Input: part model. Units: mm. Frame: model coordinates. A direction names the side the tool comes from. Coordinates: 2 decimals unless noted, no trailing zeros. Write each loop counter-clockwise with the first axis right and the second up, starting at its lowest first coordinate (ties: lowest second). Pieces come first, ordered by that corner, then holes.
from build123d import *

# Parameters (mm, degrees)
F0_W      = 14
F0_H      = 3
F0_W_2    = 3
F1_DEPTH  = 20
F2_DEPTH  = 3
F3_W      = 3
F3_H      = 3
F4_DEPTH  = 100
F5_W      = 3
F5_H      = 3.5
F6_DEPTH  = 100
F7_R      = 1.5
F9_DEPTH  = 1
F10_DEPTH = 1


with BuildPart() as f1:
    # F0 (on Front) → F1 (new body)
    with BuildSketch(Plane.XZ):
        Polygon((10, 1.5), (10, 4.5), (-10, 4.5), (-10, 1.5), (-7, 1.5), (7, 1.5), align=None)
        Rectangle(F0_W, F0_H)
        with Locations((11.5, 0)):
            Rectangle(F0_W_2, F0_H)
        with Locations((8.5, 0)):
            Rectangle(F0_W_2, F0_H)
        with Locations((-8.5, 0)):
            Rectangle(F0_W_2, F0_H)
        Polygon((10, -4.5), (10, -1.5), (7, -1.5), (-7, -1.5), (-10, -1.5), (-10, -4.5), align=None)
    extrude(amount=-F1_DEPTH)

    # F0 (on Front) → F2 (join)
    with BuildSketch(Plane.XZ):
        with Locations((-8.5, 0)):
            Rectangle(F0_W_2, F0_H)
        Rectangle(F0_W, F0_H)
        with Locations((8.5, 0)):
            Rectangle(F0_W_2, F0_H)
        with Locations((11.5, 0)):
            Rectangle(F0_W_2, F0_H)
    extrude(amount=F2_DEPTH)

    # F3 (on face) → F4 (cut)
    with BuildSketch(Plane.YZ.offset(13)):
        Polygon((23, -1.75), (23, 1.75), (17, 1.75), (17, 1.5), (20, 1.5), (20, -1.5), (17, -1.5), (17, -1.75), align=None)
        with Locations((18.5, 0)):
            Rectangle(F3_W, F3_H)
    extrude(amount=-F4_DEPTH, mode=Mode.SUBTRACT)

    # F5 (on face) → F6 (cut)
    with BuildSketch(Plane(origin=(0, 17, 0), x_dir=(-1, 0, 0), z_dir=(0, 1, 0))):
        with Locations((11.5, 0)):
            Rectangle(F5_W, F5_H)
        with Locations((8.5, 0)):
            Rectangle(F5_W, F5_H)
    extrude(amount=-F6_DEPTH, mode=Mode.SUBTRACT)

    # F7
    f7_edges = [f1.edges().sort_by_distance(p)[0] for p in [
        (-7, -3, 0),
        (13, -3, 0),
        (10, 0, 3),
        (10, 0, -3),
        (-10, 0, -3.125),
        (-10, 0, 3.125),
        (-7, 17, 0),
        (-10, 20, 3.125),
        (-10, 20, -3.125),
        (13, 17, 0),
        (10, 20, 3.125),
        (10, 20, -3.125),
    ]]
    fillet(f7_edges, radius=F7_R)

    # F8 (on face) → F9 (cut)
    with BuildSketch(Plane.XY.offset(4.5)):
        with BuildLine():
            add(Edge.make_bspline(
                [(1.6788760671, 6), (1.5308734468, 4.4721571739), (0.7623540077, 3.5911458333)],
                knots=[0.1925814922, 0.1925814922, 0.1925814922, 1, 1, 1], degree=2))
            Line((1.6788760671, 6), (-0.8607862189, 6))
            add(Edge.make_bspline(
                [(-1.1673334923, 5.1341145833), (-0.9450911222, 5.4549517504), (-0.8607862189, 6)],
                knots=[0, 0, 0, 0.6206623282, 0.6206623282, 0.6206623282], degree=2))
            add(Edge.make_bspline(
                [(-2.3561355757, 4.6171875), (-1.525406409, 4.6171875), (-1.1673334923, 5.1341145833)],
                knots=[0, 0, 0, 1, 1, 1], degree=2))
            add(Edge.make_bspline(
                [(-3.5436355757, 4.7786458333), (-2.892593909, 4.6171875), (-2.3561355757, 4.6171875)],
                knots=[0, 0, 0, 1, 1, 1], degree=2))
            Line((-3.5436355757, 4.7786458333), (-3.5436355757, 2.6796875))
            add(Edge.make_bspline(
                [(-2.0540522423, 2.5), (-2.908218909, 2.5), (-3.5436355757, 2.6796875)],
                knots=[0, 0, 0, 1, 1, 1], degree=2))
            add(Edge.make_bspline(
                [(0.7623540077, 3.5911458333), (-0.189468909, 2.5), (-2.0540522423, 2.5)],
                knots=[0, 0, 0, 1, 1, 1], degree=2))
        make_face()
    extrude(amount=-F9_DEPTH, mode=Mode.SUBTRACT)

    # F8 (on face) → F10 (cut)
    with BuildSketch(Plane.XY.offset(4.5)):
        with BuildLine():
            Line((-0.8607862189, 6), (1.6788760671, 6))
            add(Edge.make_bspline(
                [(1.7141769243, 6.765625), (1.7141769243, 6.364413558), (1.6788760671, 6)],
                knots=[0, 0, 0, 0.1925814922, 0.1925814922, 0.1925814922], degree=2))
            Line((1.7141769243, 6.765625), (1.7141769243, 17.8984375))
            Line((1.7141769243, 17.8984375), (-0.8092605757, 17.8984375))
            Line((-0.8092605757, 17.8984375), (-0.8092605757, 6.75))
            add(Edge.make_bspline(
                [(-0.8607862189, 6), (-0.8092605757, 6.3331237045), (-0.8092605757, 6.75)],
                knots=[0.6206623282, 0.6206623282, 0.6206623282, 1, 1, 1], degree=2))
        make_face()
    extrude(amount=-F10_DEPTH, mode=Mode.SUBTRACT)


solid = f1.part
Item 1: Pull-direction query (Z, two-part tool) for faces 4 (the face through (-7.4, 12.9, -1.75)), 5 (the face through (1.714, 12, 4)), 6 (the face through (5.9, -0.4, -1.5)); classes: released by +Z, released by -Z, zero draft, split by the parting line, or undercut.
Item 2: Material intervals for line 1 (Z direction, x = -0.25, y = 17.5); line 2 (Y direction, x = -2.25, z = 4); line 3 (Z direction, x = 9.5, y = 17.5), sorted ascending.
Item 3: Section query A-A, the plane x = 6. Return loops of the section in (y, z).
Item 4: Section query B-B, the plane z = 2.5. Return loops of the section in (x, y), then the cut area to 3 significant figures.
Item 5: Section query C-C, the plane y = 12.75. Return loops of the section in (x, z).
Item 6: Pin query (flat end, axial travel): pin 1 Ø4 at (y, z) = (10.5, 0) entering from -X; pin 2 Ø0.5 at (x, z) = (0, 4) entering from -Y; pin 3 Ø2 at (y, z) = (17.5, -1.5) entering from +X; pin 4 Ø1.1 at (y, z) = (11, 4) entering from +X. Return the tip coordinate at first contact, or that it passes through.
Item 7: Section query D-D, the plane y = 16. Return loops of the section in (x, z), then the cut area to 3 significant figures.
Item 8: Access query for faces 1 (the face through (-6.55, 16.57, 0.02)), 2 (the face through (0, 0, -3)), 3 (the face through (-0.809, 12, 4)). Directions: +Z, -Z, +X, -X, +Y, -Y. A direction counts if a zero-diameter tool reaches every point of the face in a straight line with its end or side. Return the directions, or none.
The answers:
1. face 4: undercut
1. face 5: zero draft
1. face 6: released by -Z
2. line 1: z = -4.5 to -1.75, 1.75 to 3.5
2. line 2: y = 0 to 2.5, 4.62 to 20
2. line 3: z = -4.5 to -1.75, 1.75 to 4.5
3. outline: (-3, -1.5) - (0, -1.5) - (0, -4.5) - (20, -4.5) - (20, -1.75) - (17, -1.75) - (17, 1.75) - (20, 1.75) - (20, 4.5) - (0, 4.5) - (0, 1.5) - (-3, 1.5) - close
4. outline: (-10, 1.5) arc R1.5 ccw to (-8.5, 0) - (8.5, 0) arc R1.5 ccw to (10, 1.5) - (10, 18.5) arc R1.5 ccw to (8.5, 20) - (-8.5, 20) arc R1.5 ccw to (-10, 18.5) - close
4. area: 398 mm2
5. outline: (-10, -4.5) - (10, -4.5) - (10, -1.5) - (13, -1.5) - (13, 1.5) - (10, 1.5) - (10, 4.5) - (1.71, 4.5) - (1.71, 3.5) - (-0.81, 3.5) - (-0.81, 4.5) - (-10, 4.5) - (-10, 1.75) - (-7, 1.75) - (-7, -1.75) - (-10, -1.75) - close
6. pin 1: stops at x = -10
6. pin 2: stops at y = 0
6. pin 3: stops at x = 12.62
6. pin 4: stops at x = 10
7. outline: (-10, -4.5) - (10, -4.5) - (10, -1.5) - (12.91, -1.5) - (12.91, 1.5) - (10, 1.5) - (10, 4.5) - (1.71, 4.5) - (1.71, 3.5) - (-0.81, 3.5) - (-0.81, 4.5) - (-10, 4.5) - (-10, 1.75) - (-6.91, 1.75) - (-6.91, -1.75) - (-10, -1.75) - close
7. area: 175 mm2
8. face 1: -X, +Y
8. face 2: -Z, +X, -X, -Y
8. face 3: +Z
